```python
from build123d import *

# Parameters (mm, degrees)
SKETCH2_R           = 12.7
BOSS_EXTRUDE1_DEPTH = 1.27
SKETCH3_R           = 3.175
BOSS_EXTRUDE2_DEPTH = 6.35
CIRPATTERN1_COUNT   = 3
CHAMFER1_SIZE       = 5.08
CHAMFER1_SIZE2      = 2.932939367
CHAMFER2_SIZE       = 5.08
CHAMFER2_SIZE2      = 2.156332066
CHAMFER3_SIZE       = 5.08
CHAMFER3_SIZE2      = 1.45666656
FILLET1_R           = 2.54


with BuildPart() as part:
    # Sketch2 → Boss-Extrude1 (new body)
    with BuildSketch(Plane(origin=(0, 0, 0), x_dir=(1, 0, 0), z_dir=(0, 1, 0))):
        with Locations(Location((0, 0, 0), (0, 0, 270))):
            Circle(SKETCH2_R)
    extrude(amount=BOSS_EXTRUDE1_DEPTH)

    # Sketch3 → Boss-Extrude2 (add)
    with BuildSketch(Plane.XZ):
        with Locations(Location((0, 7.62, 0), (0, 0, 270))):
            Circle(SKETCH3_R)
    boss_extrude2 = extrude(amount=BOSS_EXTRUDE2_DEPTH)

    # CirPattern1: Boss-Extrude2 ×3 about axis
    cirpattern1_axis = Axis((0, 0, 0), (0, 1, 0))
    for i in range(1, CIRPATTERN1_COUNT):
        add(boss_extrude2.rotate(cirpattern1_axis, i * 360 / CIRPATTERN1_COUNT))

    # Chamfer1
    chamfer1_edges = [part.edges().sort_by_distance(p)[0] for p in [
        (0, -6.35, 10.795),
    ]]
    chamfer1_side = [part.faces().sort_by_distance(p)[0] for p in [
        (0, -3.175, 10.795),
    ]]
    chamfer(chamfer1_edges, length=CHAMFER1_SIZE, length2=CHAMFER1_SIZE2, reference=chamfer1_side[0])

    # Chamfer2
    chamfer2_edges = [part.edges().sort_by_distance(p)[0] for p in [
        (9.348744234, -6.35, -5.3975),
    ]]
    chamfer2_side = [part.faces().sort_by_distance(p)[0] for p in [
        (9.348744234, -3.175, -5.3975),
    ]]
    chamfer(chamfer2_edges, length=CHAMFER2_SIZE, length2=CHAMFER2_SIZE2, reference=chamfer2_side[0])

    # Chamfer3
    chamfer3_edges = [part.edges().sort_by_distance(p)[0] for p in [
        (-9.348744234, -6.35, -5.3975),
    ]]
    chamfer3_side = [part.faces().sort_by_distance(p)[0] for p in [
        (-9.348744234, -3.175, -5.3975),
    ]]
    chamfer(chamfer3_edges, length=CHAMFER3_SIZE, length2=CHAMFER3_SIZE2, reference=chamfer3_side[0])

    # Fillet1
    fillet1_edges = [part.edges().sort_by_distance(p)[0] for p in [
        (0, -1.27, 10.795),
        (9.348744234, -1.27, -5.3975),
        (-9.348744234, -1.27, -5.3975),
    ]]
    fillet(fillet1_edges, radius=FILLET1_R)


solid = part.part
```
Could you check a few things on this model? Use its own coordinates, in mm. A direction names the side the tool comes from. Round coordinates to 2 decimals unless told otherwise and drop trailing zeros. Loops run counter-clockwise (first coordinate to the right, second up) from the corner with the lowest first, then second, coordinate; pieces in that order, holes last. Notation, with made-up numbers: (1.25, 21.25) -> (58.25, 21.25) arc R24 ccw to (58.25, 40.25) -> close; hole circle Ø2 at (57.25, 17). An arc over 180 degrees is marked (long way). One line per question, with ' | ' between items.
(1) Thinking about a two-plate mould opening in X: for faces 3 (the face through (5.38, -0.37, -6.74)), 4 (the face through (0.14, -0.29, 10.79)), 5 (the face through (-7, -6.35, -4)), which applies, released by +X, released by -X, zero draft, split by the parting line, or undercut?
Model answer:
face 3: undercut | face 4: split by the parting line | face 5: zero draft
(2) If we section it at A-A on y = -3: List the corners of the cut face in (x, z) for me, and give its area (3 significant figures).
Model answer:
outline: circle Ø5.36 at (-6.6, -3.81); circle Ø4.35 at (0, 7.62); circle Ø4.88 at (6.6, -3.81) | area: 56.1 mm^2
(3) For pin 1 Ø3 at (y, z) = (-2.5, -7) entering from +X; pin 2 Ø1 at (x, z) = (-0.5, -1.5) entering from -Y; pin 3 Ø4 at (x, y) = (-3, -3) entering from -Z, each with a flat end and sliding along its axis, tell me the tip position at first contact or that it passes through.
Model answer:
pin 1: stops at x = 8.89 | pin 2: stops at y = 0 | pin 3: stops at z = -6.12
(4) For faces 1 (the face through (-3.922, -0.45, -5.517)), 2 (the face through (-7.7, 0.6, -10.1)), which set-ups out of +Z, -Z, +X, -X, +Y, -Y let a thin tool reach every point of the face, with its end or its side?
Model answer:
face 1: -Y | face 2: +Y, -Y
(5) If we section it at B-B on z = 1: List the corners of the cut face in (x, y) for me, and give its area (3 significant figures).
Model answer:
outline: (-12.66, 0) -> (12.66, 0) -> (12.66, 1.27) -> (-12.66, 1.27) -> close | area: 32.2 mm^2
(6) If I drill on probe 1 along Y at (x, z) = (-8, 9); probe 2 along X at (y, z) = (-1.25, -4); probe 3 along X at (y, z) = (-2, 6), over which ranges is the centre line in solid material (lowest first)?
Model answer:
probe 1: y = 0 to 1.27 | probe 2: x = -9.75 to -3.45, 3.48 to 9.72 | probe 3: x = -2.23 to 2.23
